Work out the finished part from the listing and answer in its coordinate system (mm). A direction names the side the tool comes from. Round coordinates to 2 decimals unless told otherwise and drop trailing zeros. Loops run counter-clockwise (first coordinate to the right, second up) from the corner with the lowest first, then second, coordinate; pieces in that order, holes last. Notation, with made-up numbers: (66, 43.25) - (123, 43.25) arc R28 cw to (123, 67.25) - close; hole circle Ø5 at (72, -4). An arc over 180 degrees is marked (long way). Use CSV: the item, a comma, the result in double quotes. Start each with the question number.
Autodesk Fusion 360 part; units mm, degrees
sketch "Sketch1" plane through (0, 0, 0) normal (0, 0, 1) x (1, 0, 0)
  line L0 (-7.8581, 65) -> (-7.8581, 62)
  circle A0 centre (-40, 7) radius 2.5
  line L1 (-32.5, 22) -> (32.5, 22) construction
  line L2 (-40, 61) -> (-40, 7) construction
  arc A1 (19, 8) -> (15, 12) centre (15, 8) ccw
  line L3 (40, 7) -> (40, 61) construction
  arc A2 (-7.8581, 65) -> (-11.7311, 68) centre (-11.7311, 64) ccw
  arc A3 (-50, 4) -> (-46, 0) centre (-46, 4) ccw
  arc A4 (50, 64) -> (46, 68) centre (46, 64) ccw
  line L4 (19, 4) -> (19, 8)
  line L5 (7.8581, 65) -> (7.8581, 62)
  line L6 (-11.7311, 68) -> (-46, 68)
  circle A5 centre (32.5, 22) radius 3.6
  line L7 (-40, 7) -> (40, 7) construction
  line L8 (-30, 41) -> (30, 41) construction
  circle A6 centre (40, 61) radius 2.5
  circle A7 centre (40, 7) radius 2.5
  arc A8 (19, 4) -> (23, 0) centre (23, 4) ccw
  arc A9 (-46, 68) -> (-50, 64) centre (-46, 64) ccw
  line L9 (0, 0) -> (0, 50.832) construction
  arc A10 (11.7311, 68) -> (7.8581, 65) centre (11.7311, 64) ccw
  arc A11 (-15, 12) -> (-19, 8) centre (-15, 8) ccw
  line L10 (-50, 64) -> (-50, 4)
  arc A12 (-7.8581, 62) -> (7.8581, 62) centre (0, 63.5) ccw
  line L11 (15, 12) -> (-15, 12)
  circle A13 centre (-32.5, 22) radius 3.6
  arc A14 (-23, 0) -> (-19, 4) centre (-23, 4) ccw
  line L12 (23, 0) -> (46, 0)
  line L13 (46, 68) -> (11.7311, 68)
  line L14 (-50, 34) -> (50, 34) construction
  circle A15 centre (-30, 41) radius 2.5
  circle A16 centre (-40, 61) radius 2.5
  line L15 (40, 61) -> (-40, 61) construction
  line L16 (50, 4) -> (50, 64)
  arc A17 (46, 0) -> (50, 4) centre (46, 4) ccw
  line L17 (-19, 8) -> (-19, 4)
  line L18 (-46, 0) -> (-23, 0)
  circle A18 centre (30, 41) radius 2.5
  point P0 (-50, 68)
  point P1 (-50, 0)
  point P2 (-50, 0)
  dimension "d1" = 68
  dimension "d3" = 50
  dimension "d4" = 19
  dimension "d5" = 19
  dimension "d6" = 40
  dimension "d7" = 40
  dimension "d8" = 50
  dimension "d9" = 32.5
  dimension "d10" = 32.5
  dimension "d11" = 30
  dimension "d13" = 54
  dimension "d14" = 27
  dimension "d15" = 7
  dimension "d16" = 12
  dimension "d17" = 4
  dimension "d18" = 4
  dimension "d19" = 4
  dimension "d20" = 4
  dimension "d24" = 8
  dimension "d25" = 4.5
  dimension "d27" = 6
  dimension "d28" = 3
  dimension "d29" = 4
  dimension "d30" = 6
  dimension "d32" = 4
  dimension "d35" = 50
  dimension "d36" = 4
  dimension "d37" = 4
  dimension "d38" = 30
  dimension "d39" = 15
  dimension "d40" = 34
  dimension "d44" = 12
  dimension "d45" = 7.2
  dimension "d46" = 5
  dimension "d47" = 30
  dimension "d47" = 30
extrude "Extrude1" add sketch "Sketch1" along normal blind 4
equation "d4 = ( 38 / 2 ) * 1 mm"
equation "d9 = ( 65 / 2 ) * 1 mm"
equation "d14 = ( 54 / 2 ) * 1 mm"
Item 1: A cutting plane is placed at B-B (z = 2.7). State how many separate pieces and enclosed holes the cut face has, plus the area to 3 significant figures.
Item 2: A cutting plane is placed at D-D (y = 7). Determine the outline of the cut face in (x, z), plus the area to 3 significant figures.
Item 3: A cutting plane is placed at C-C (x = -40). Determine the outline of the cut face in (y, z).
Item 4: Find the intervals of material crossed by probe 1 along X at (y, z) = (43, 3.5); probe 2 along Y at (x, z) = (30, 3); probe 3 along X at (y, z) = (9, 3.2), in increasing order. Write a range as [from, to].
Item 5: Which of the six approach directions +Z, -Z, +X, -X, +Y, -Y give full straight-line access (tool end or side, diameter ignored) to faces 1 (the cylindrical face through (20.203, 1.141, 1.972)), 2 (the cylindrical face through (29.46, 43.44, 1.97))?
Item 6: The mould has two halves that part along X. Classify faces 3 (the cylindrical face through (48.797, 66.859, 1.972)), 4 (the cylindrical face through (-48.797, 1.141, 1.972)), 5 (the flat face through (-1, 34, 0)), 6 (the flat face through (-7.858, 64, 2)): pulls with the +X half, pulls with the -X half, needs draft (parallel to the pull), parting line crosses it, or undercut.
Item 7: A cutting plane is placed at A-A (y = 22). Determine the outline of the cut face in (x, z), plus the area to 3 significant figures.
Item 8: Each of these flat-tipped pins is pushed along its axis until it touches: pin 1 Ø4 at (x, y) = (40, 7) entering from -Z; pin 2 Ø1.2 at (x, z) = (2, 2) entering from -Y. Where does it stop, or does it pass through?
Result sheet:
1,separate pieces,"1"
1,enclosed holes,"8"
1,area,"5,950 mm^2"
2,outline,"(-50, 0) - (-42.5, 0) - (-42.5, 4) - (-50, 4) - close; (-37.5, 0) - (-19, 0) - (-19, 4) - (-37.5, 4) - close; (19, 0) - (37.5, 0) - (37.5, 4) - (19, 4) - close; (42.5, 0) - (50, 0) - (50, 4) - (42.5, 4) - close"
2,area,"208 mm^2"
3,outline,"(0, 0) - (4.5, 0) - (4.5, 4) - (0, 4) - close; (9.5, 0) - (58.5, 0) - (58.5, 4) - (9.5, 4) - close; (63.5, 0) - (68, 0) - (68, 4) - (63.5, 4) - close"
4,probe 1,"[-50, -31.5], [-28.5, 28.5], [31.5, 50]"
4,probe 2,"[0, 19.41], [24.59, 38.5], [43.5, 68]"
4,probe 3,"[-50, -41.5], [-38.5, -18.87], [18.87, 38.5], [41.5, 50]"
5,face 1,"+Z, -Z, -Y"
5,face 2,"+Z, -Z"
6,face 3,"pulls with the +X half"
6,face 4,"pulls with the -X half"
6,face 5,"needs draft"
6,face 6,"undercut"
7,outline,"(-50, 0) - (-36.1, 0) - (-36.1, 4) - (-50, 4) - close; (-28.9, 0) - (28.9, 0) - (28.9, 4) - (-28.9, 4) - close; (36.1, 0) - (50, 0) - (50, 4) - (36.1, 4) - close"
7,area,"342 mm^2"
8,pin 1,"through"
8,pin 2,"y = 12"
